Build history of the part. All positions in model axes, mm. A direction names the side the tool comes from. Coordinates: 2 decimals unless noted, no trailing zeros. Loops run counter-clockwise (first coordinate to the right, second up) from the corner with the lowest first, then second, coordinate; pieces in that order, holes last. Notation, with made-up numbers: (23, 9.25) - (40, 9.25) arc R22 cw to (40, 46.25) - close; hole circle Ø4 at (87, 18.25). An arc over 180 degrees is marked (long way). One line per item, written item: value.
Autodesk Fusion 360 part; units mm, degrees
sketch "Sketch1" plane through (0, 0, 0) normal (0, 1, 0) x (1, 0, 0)
  circle A0 centre (0, 0) radius 13 construction
  circle A1 centre (0, 0) radius 11.8004
  point P0 (-7.45, 0.5)
  point P1 (-7.45, -0.75)
  point P2 (-7.4065, -2.039)
  point P3 (9.3586, 0.2369)
  point P4 (9.3586, -0.9412)
  point P5 (8.3, -3.7)
  point P6 (-4.8, -8.9)
  point P7 (-0.0017, -8.7426)
  point P8 (4.1864, -8.1521)
  point P9 (2.9094, -8.1521)
  point P10 (3.1291, -9.6832)
  dimension "d1" = 26
extrude "Extrude1" add sketch "Sketch1" against normal blind 2
hole "Hole1" at (-7.45, 0, -0.5) at (-7.45, 0, 0.75) at (-7.4065, 0, 2.039) at (-4.8, 0, 8.9) at (-0.0017, 0, 8.7426) at (2.9094, 0, 8.1521) at (3.1291, 0, 9.6832) at (4.1864, 0, 8.1521) at (8.3, 0, 3.7) at (9.3586, 0, 0.9412) at (9.3586, 0, -0.2369) direction (0, -1, 0) diameter 1.6 depth 5.5 tip angle 118
hole "Hole2" at (0, 0, 0) direction (0, -1, 0) diameter 3.5 depth 5.5 tip angle 118
Item 1: Cut at C-C, the plane z = 3.7. Write the cut outline in (x, y), then the cut area to 3 significant figures.
Check result:
outline: (-11.21, -2) - (7.5, -2) - (7.5, 0) - (-11.21, 0) - close; (9.1, -2) - (11.21, -2) - (11.21, 0) - (9.1, 0) - close
area: 41.6 mm^2
Item 2: Cut at B-B, the plane x = -4.8. Write the cut outline in (y, z), then the cut area to 3 significant figures.
Check result:
outline: (-2, -10.78) - (0, -10.78) - (0, 8.1) - (-2, 8.1) - close; (-2, 9.7) - (0, 9.7) - (0, 10.78) - (-2, 10.78) - close
area: 39.9 mm^2
Item 3: Tool access for faces 4 (the face through (2, -2, 0)), 5 (the face through (-8.25, -1.01, 0.79)): list every direction of +Z, -Z, +X, -X, +Y, -Y with a clear straight run to the whole face (end or side of a thin tool).
Check result:
face 4: +Z, -Z, +X, -X, -Y
face 5: +Y, -Y
Item 4: Cut at D-D, the plane y = -1.15. Give the number of separate pieces and of enclosed holes in the cut face, then the cut area to 3 significant figures.
Check result:
separate pieces: 1
enclosed holes: 7
area: 407 mm^2
Item 5: Probe probe 1 along X at (y, z) = (-0.8, 9); probe 2 along X at (y, z) = (-1.45, -0.5); probe 3 along Z at (x, y) = (3.5, -0.6). List the from-to ranges inside material, lowest first. Write a range as from..to.
Check result:
probe 1: x = -7.63..-5.59, -4.01..-0.76, 0.76..2.71, 3.55..7.63
probe 2: x = -11.79..-8.25, -6.65..-1.68, 1.68..8.6, 10.11..11.79
probe 3: z = -11.27..7.61, 8.69..8.97, 10.39..11.27
Item 6: Cut at A-A, the plane z = -0.5. Write the cut outline in (x, y).
Check result:
outline: (-11.79, -2) - (-8.25, -2) - (-8.25, 0) - (-11.79, 0) - close; (-6.65, -2) - (-1.68, -2) - (-1.68, 0) - (-6.65, 0) - close; (1.68, -2) - (8.6, -2) - (8.6, 0) - (1.68, 0) - close; (10.11, -2) - (11.79, -2) - (11.79, 0) - (10.11, 0) - close
Item 7: Pull direction X, two halves, no side cores. Call faces 1 (the face through (-6.65, -1.01, 0.74)), 2 (the face through (-2.56, -0.99, 11.52)), 3 (the face through (2, 0, 0)): released by +X, released by -X, zero draft, split by the parting line, or undercut.
Check result:
face 1: undercut
face 2: split by the parting line
face 3: zero draft
